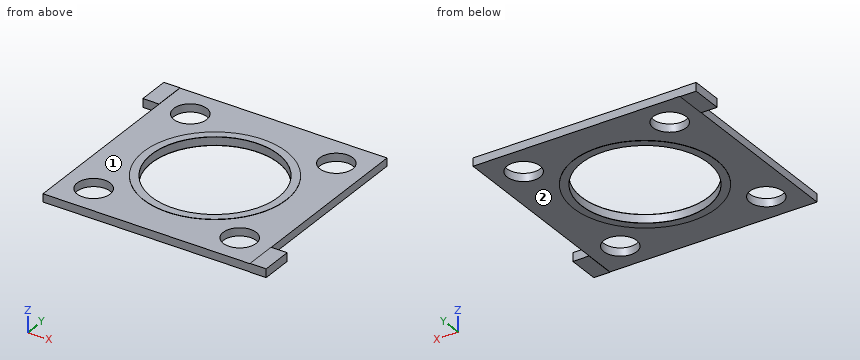
```python
from build123d import *

# Parameters (mm, degrees)
SKETCH1_W                = 41.402
SKETCH1_H                = 41.402
BOSS_EXTRUDE1_DEPTH      = 0.79883
BOSS_EXTRUDE1_DEPTH_BACK = 0.79883
SKETCH2_W                = 3.22834
SKETCH2_H                = 6.35
BOSS_EXTRUDE2_DEPTH      = 0.79883
BOSS_EXTRUDE2_DEPTH_BACK = 0.79883
SKETCH3_R                = 12.7
CUT_EXTRUDE1_DEPTH       = 2.59766
SKETCH4_R                = 14.2875
SKETCH4_R_2              = 12.7
BOSS_EXTRUDE3_DEPTH      = 0.0508
SKETCH5_W                = 3.22834
SKETCH5_H                = 6.35
BOSS_EXTRUDE4_DEPTH      = 0.0508
SKETCH6_R                = 3.302
CUT_EXTRUDE2_DEPTH       = 2.64846


with BuildPart() as part:
    # Sketch1 → Boss-Extrude1 (new body, two sides)
    with BuildSketch(Plane.XY) as boss_extrude1_sk:
        Rectangle(SKETCH1_W, SKETCH1_H)
    extrude(amount=BOSS_EXTRUDE1_DEPTH)
    extrude(boss_extrude1_sk.sketch, amount=-BOSS_EXTRUDE1_DEPTH_BACK)

    # Sketch2 → Boss-Extrude2 (add, two sides)
    with BuildSketch(Plane.XY) as boss_extrude2_sk:
        with Locations((-22.31517, 17.526)):
            Rectangle(SKETCH2_W, SKETCH2_H)
        with Locations((22.31517, -17.526)):
            Rectangle(SKETCH2_W, SKETCH2_H)
    extrude(amount=BOSS_EXTRUDE2_DEPTH)
    extrude(boss_extrude2_sk.sketch, amount=-BOSS_EXTRUDE2_DEPTH_BACK)

    # Sketch3 → Cut-Extrude1 (cut, through all)
    with BuildSketch(Plane.XY.offset(0.79883)):
        Circle(SKETCH3_R)
    extrude(amount=-CUT_EXTRUDE1_DEPTH, mode=Mode.SUBTRACT)

    # Sketch4 → Boss-Extrude3 (add)
    with BuildSketch(Plane.XY.offset(0.79883)):
        Circle(SKETCH4_R)
        Circle(SKETCH4_R_2, mode=Mode.SUBTRACT)
    boss_extrude3 = extrude(amount=BOSS_EXTRUDE3_DEPTH)

    # Sketch5 → Boss-Extrude4 (add)
    with BuildSketch(Plane.XY.offset(0.79883)):
        with Locations((-22.31517, 17.526)):
            Rectangle(SKETCH5_W, SKETCH5_H)
        with Locations((22.31517, -17.526)):
            Rectangle(SKETCH5_W, SKETCH5_H)
    boss_extrude4 = extrude(amount=BOSS_EXTRUDE4_DEPTH)

    # Mirror3: Boss-Extrude3, Boss-Extrude4 across plane
    add(boss_extrude3.mirror(Plane.XY))
    add(boss_extrude4.mirror(Plane.XY))

    # Sketch6 → Cut-Extrude2 (cut, through all)
    with BuildSketch(Plane.XY.offset(0.79883)):
        with Locations((-14.605, 14.605)):
            Circle(SKETCH6_R)
        with Locations((14.605, 14.605)):
            Circle(SKETCH6_R)
    cut_extrude2 = extrude(amount=-CUT_EXTRUDE2_DEPTH, mode=Mode.SUBTRACT)

    # Mirror4: Cut-Extrude2 across plane
    add(cut_extrude2.mirror(Plane.ZX), mode=Mode.SUBTRACT)


solid = part.part
```
The listing builds one solid part. Answer for the finished solid, in the listing's coordinates (mm). Face numbers are marked on the shaded views. A direction names the side the tool comes from. Coordinates: 2 decimals unless noted, no trailing zeros. Write each loop counter-clockwise with the first axis right and the second up, starting at its lowest first coordinate (ties: lowest second). Pieces come first, ordered by that corner, then holes. Notation, with made-up numbers: (41, 33) - (98, 33) arc R29 cw to (98, 69) - close; hole circle Ø1 at (-14.75, 19.25). An arc over 180 degrees is marked (long way). Return JSON: item names as keys, results as strings. Group by question number.
1. A cutting plane is placed at A-A, the plane x = 0. Determine the outline of the cut face in (y, z).
2. A cutting plane is placed at C-C, the plane y = -16.5. Determine the outline of the cut face in (x, z), plus the area to 3 significant figures.
3. Given pin 1 (8.5 mm diameter, centred on x = -14.605, y = 14.605, fed in from +Z); pin 2 (0.5 mm diameter, centred on y = 6, z = 0.5, fed in from +X), each flat-ended and moving along its own axis, determine where each tip first touches the part or whether it passes through.
4. Straight lines are drawn through the part: L1, parallel to X at y = -0.5, z = -0.45; L2, parallel to X at y = -14, z = 0.3; L3, parallel to X at y = -17, z = 0. For each, find the intervals that lie inside material, in ascending order.
5. Which of the six approach directions +Z, -Z, +X, -X, +Y, -Y give full straight-line access (tool end or side, diameter ignored) to the marked faces 1 and 2?
6. A cutting plane is placed at D-D, the plane x = -16.5. Determine the outline of the cut face in (y, z), plus the area to 3 significant figures.
Ans:
{
 "1": {"outline": "(-20.7, -0.8) - (-14.29, -0.8) - (-14.29, -0.85) - (-12.7, -0.85) - (-12.7, 0.85) - (-14.29, 0.85) - (-14.29, 0.8) - (-20.7, 0.8) - close; (12.7, -0.85) - (14.29, -0.85) - (14.29, -0.8) - (20.7, -0.8) - (20.7, 0.8) - (14.29, 0.8) - (14.29, 0.85) - (12.7, 0.85) - close"},
 "2": {"outline": "(-20.7, -0.8) - (-17.31, -0.8) - (-17.31, 0.8) - (-20.7, 0.8) - close; (-11.9, -0.8) - (11.9, -0.8) - (11.9, 0.8) - (-11.9, 0.8) - close; (17.31, -0.8) - (20.7, -0.8) - (20.7, -0.85) - (23.93, -0.85) - (23.93, 0.85) - (20.7, 0.85) - (20.7, 0.8) - (17.31, 0.8) - close", "area": "54.4 mm²"},
 "3": {"pin 1": "z = 0.8", "pin 2": "x = 20.7"},
 "4": {"L1": "-20.7 to -12.69, 12.69 to 20.7", "L2": "-20.7 to -17.85, -11.36 to 11.36, 17.85 to 20.7", "L3": "-20.7 to -16.88, -12.33 to 12.33, 16.88 to 23.93"},
 "5": {"face 1": "+Z", "face 2": "-Z"},
 "6": {"outline": "(-20.7, -0.8) - (-17.31, -0.8) - (-17.31, 0.8) - (-20.7, 0.8) - close; (-11.9, -0.8) - (11.9, -0.8) - (11.9, 0.8) - (-11.9, 0.8) - close; (17.31, -0.8) - (20.7, -0.8) - (20.7, 0.8) - (17.31, 0.8) - close", "area": "48.9 mm²"}
}
